```python
from build123d import *

# Parameters (mm, degrees)
SKETCH3_R           = 198.4375
BOSS_EXTRUDE1_DEPTH = 1.5875


with BuildPart() as part:
    # Sweep1: sweep along a path in Sketch1
    with BuildLine(Plane(origin=(0, 0, 0), x_dir=(1, 0, 0), z_dir=(0, 1, 0))) as sweep1_path:
        CenterArc((0, 0), 196.85, 0, 360)
    # Sketch2 → Sweep1 (sweep)
    with BuildSketch(Plane.XY):
        Polygon((196.85, 0), (196.85, 762), (203.2, 762), (203.2, 749.3), (201.6125, 749.3), (201.6125, 760.4125), (198.4375, 760.4125), (198.4375, 0), align=None)
    sweep(path=sweep1_path.line)

    # Sketch3 → Boss-Extrude1 (add)
    with BuildSketch(Plane(origin=(0, 0, 0), x_dir=(-1, 0, 0), z_dir=(0, -1, 0))):
        with Locations(Location((0, 0, 0), (0, 0, 180))):
            Circle(SKETCH3_R)
    extrude(amount=BOSS_EXTRUDE1_DEPTH)

    # Fillet1: read off the stored shape, not the designer's step
    # Fillet1 outline → Fillet1 (revolve, cut)
    with BuildSketch(Plane.XY):
        with BuildLine():
            Line((196.85, 762), (196.85, 759.46))
            ThreePointArc((196.85, 759.46), (197.593948776, 761.256051224), (199.39, 762))
            Line((199.39, 762), (196.85, 762))
        make_face()
        with BuildLine():
            Line((198.4375, -1.5875), (198.4375, 0.9525))
            ThreePointArc((198.4375, 0.9525), (197.693551224, -0.843551224), (195.8975, -1.5875))
            Line((195.8975, -1.5875), (198.4375, -1.5875))
        make_face()
    revolve(axis=Axis((0, 0, 0), (0, 1, 0)), mode=Mode.SUBTRACT)


solid = part.part
```
Input: part model. Units: mm. Frame: model coordinates. A direction names the side the tool comes from. Coordinates: 2 decimals unless noted, no trailing zeros. Answer as a JSON object with one key per item and string values.
1. Access query for faces 4 (the face through (187.76, 374.41, -59.13)), 5 (the face through (-43.02, 386, 193.72)). Directions: +Z, -Z, +X, -X, +Y, -Y. A direction counts if a zero-diameter tool reaches every point of the face in a straight line with its end or side. Return the directions, or none.
Result set:
{"face 4": "+Y", "face 5": "-Y"}
2. Mould query, pull axis Z, two halves, no side actions, for faces 1 (the face through (-3, -1.588, 3)), 2 (the face through (-3, 0, 3)), 3 (the face through (-44.05, 755.739, 198.368)). Classes: released by +Z, released by -Z, zero draft, split by the parting line, or undercut.
Result set:
{"face 1": "zero draft", "face 2": "undercut", "face 3": "split by the parting line"}
3. First-contact query: P1, Ø2, axis at y = 223.5, z = -7.5, coming from the +X side; P2, Ø3, axis at y = 385.5, z = -18, coming from the +X side; P3, Ø8, axis at y = 378, z = -26.5, coming from the -X side. Flat tips, straight axial feed; report the tip coordinate or a pass-through.
Result set:
{"P1": "stops at x = 198.33", "P2": "stops at x = 197.75", "P3": "stops at x = -197.16"}
4. Material intervals for line 1 (X direction, y = 485, z = 6.5); line 2 (X direction, y = 598, z = -6); line 3 (Y direction, x = -41.5, z = -39.5), sorted ascending. Write a range as from..to.
Result set:
{"line 1": "x = -198.33..-196.74, 196.74..198.33", "line 2": "x = -198.35..-196.76, 196.76..198.35", "line 3": "y = -1.59..0"}
